Source: CAD feature listing. Evaluate the final solid. Frame: model axes, mm. Give positions to 0.01 mm unless a question says otherwise; leave off trailing zeros. Loops run counter-clockwise (first coordinate to the right, second up) from the corner with the lowest first, then second, coordinate; pieces in that order, holes last. Notation, with made-up numbers: M -27.5,44 L 7.5,44 A8 cw 7.5,49 Z; hole C 0.25,-1.5 d5. An arc over 180 degrees is marked long. Put each result on its own line as item: value.
from build123d import *

# Parameters (mm, degrees)
BOSS_EXTRUDE1_DEPTH = 2
SKETCH2_R           = 1.5
CUT_EXTRUDE1_DEPTH  = 3


with BuildPart() as part:
    # Sketch1 → Boss-Extrude1 (new body)
    with BuildSketch(Plane.XY):
        with BuildLine():
            Line((-43, 260), (43, 260))
            ThreePointArc((43, 260), (50.071067812, 262.928932188), (53, 270))
            Line((53, 270), (53, 350))
            ThreePointArc((53, 350), (50.071067812, 357.071067812), (43, 360))
            Line((43, 360), (-43, 360))
            ThreePointArc((-43, 360), (-50.071067812, 357.071067812), (-53, 350))
            Line((-53, 350), (-53, 270))
            ThreePointArc((-53, 270), (-50.071067812, 262.928932188), (-43, 260))
        make_face()
    extrude(amount=-BOSS_EXTRUDE1_DEPTH)

    # Sketch2 → Cut-Extrude1 (cut)
    with BuildSketch(Plane(origin=(0, 0, -2), x_dir=(-1, 0, 0), z_dir=(0, 0, -1))):
        with Locations((47, 266)):
            Circle(SKETCH2_R)
        with Locations((47, 354)):
            Circle(SKETCH2_R)
        with Locations((-47, 354)):
            Circle(SKETCH2_R)
        with Locations((-47, 266)):
            Circle(SKETCH2_R)
    extrude(amount=-CUT_EXTRUDE1_DEPTH, mode=Mode.SUBTRACT)


solid = part.part
1. Section query B-B (y = 266). Output: boundary loops of the cut face in (x, z), plus the area to 3 significant figures.
Found:
outline: M -52.17,-2 L -48.5,-2 L -48.5,0 L -52.17,0 Z; M -45.5,-2 L 45.5,-2 L 45.5,0 L -45.5,0 Z; M 48.5,-2 L 52.17,-2 L 52.17,0 L 48.5,0 Z
area: 197 mm^2
2. Section query A-A (x = -47). Output: boundary loops of the cut face in (y, z).
Found:
outline: M 260.83,-2 L 264.5,-2 L 264.5,0 L 260.83,0 Z; M 267.5,-2 L 352.5,-2 L 352.5,0 L 267.5,0 Z; M 355.5,-2 L 359.17,-2 L 359.17,0 L 355.5,0 Z
3. Material intervals for line 1 (Y direction, x = 47, z = -0.65); line 2 (X direction, y = 354, z = -0.65), sorted ascending. Write a range as from..to.
Found:
line 1: 260.83..264.5, 267.5..352.5, 355.5..359.17
line 2: -52.17..-48.5, -45.5..45.5, 48.5..52.17
4. Draft query along Y for faces 1 (the flat face through (-1, 311, 0)), 2 (the cylindrical face through (-46.675, 352.536, -1.014)), 3 (the cylindrical face through (-49.99, 357.15, -0.99)). Return one class per face: pulls with the +Y half, pulls with the -Y half, needs draft (parallel to the pull), parting line crosses it, or undercut.
Found:
face 1: needs draft
face 2: undercut
face 3: pulls with the +Y half
5. Contact query for a flat-ended pin moving along its axis: P1, Ø2.5, axis at x = 47, y = 354, coming from the -Z side. Output: stop coordinate, or through.
Found:
P1: through
